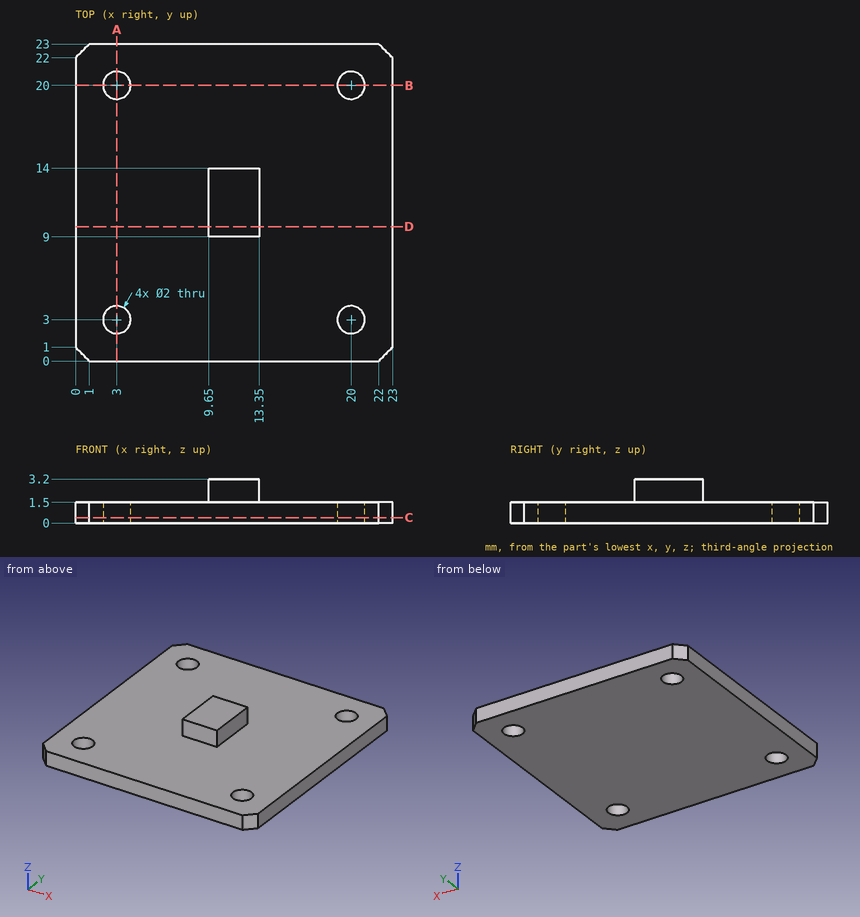
Design review of the part shown in the three views and the two pictorial views. Dimensions are in mm from the part's minimum x, y and z. Coordinates: 2 decimals unless noted, no trailing zeros. Loops run counter-clockwise (first coordinate to the right, second up) from the corner with the lowest first, then second, coordinate; pieces in that order, holes last.
Q1. We need section C-C on z = 0.4. State the section outline as (x, y) points.
Reported:
outline: (0, 1) - (1, 0) - (22, 0) - (23, 1) - (23, 22) - (22, 23) - (1, 23) - (0, 22) - close; hole circle Ø2 at (3, 3); hole circle Ø2 at (3, 20); hole circle Ø2 at (20, 3); hole circle Ø2 at (20, 20)
Q2. For pin 1 (0.8 mm diameter, centred on x = 11, z = 2.5, fed in from +Y); pin 2 (3 mm diameter, centred on x = 3, y = 3, fed in from +Z); pin 3 (0.5 mm diameter, centred on y = 11.5, z = 2.5, fed in from -X), all flat-tipped, find the tip position at first contact; note any pin that passes through.
Reported:
pin 1: stops at y = 14
pin 2: stops at z = 1.5
pin 3: stops at x = 9.65
Q3. We need section D-D on y = 9.75. State the section outline as (x, z) points, and give its area (3 significant figures).
Reported:
outline: (0, 0) - (23, 0) - (23, 1.5) - (13.35, 1.5) - (13.35, 3.2) - (9.65, 3.2) - (9.65, 1.5) - (0, 1.5) - close
area: 40.8 mm2
Q4. We need section A-A on x = 3. State the section outline as (y, z) points, and give its area (3 significant figures).
Reported:
outline: (0, 0) - (2, 0) - (2, 1.5) - (0, 1.5) - close; (4, 0) - (19, 0) - (19, 1.5) - (4, 1.5) - close; (21, 0) - (23, 0) - (23, 1.5) - (21, 1.5) - close
area: 28.5 mm2
Q5. To check wall thickness, follow line 1 (Y direction, x = 3, z = 0.55); line 2 (X direction, y = 3.75, z = 1.4). State the ranges of each line that lie inside material, in increasing order.
Reported:
line 1: y = 0 to 2, 4 to 19, 21 to 23
line 2: x = 0 to 2.34, 3.66 to 19.34, 20.66 to 23
